Here's how the part is built. I have some questions about the finished solid (model axes, mm). Round coordinates to 2 decimals unless told otherwise and drop trailing zeros. Loops run counter-clockwise (first coordinate to the right, second up) from the corner with the lowest first, then second, coordinate; pieces in that order, holes last. Notation, with made-up numbers: M 36.25,20.25 L 68.25,20.25 A16 ccw 68.25,49.25 Z; hole C 50,74.5 d3. An arc over 180 degrees is marked long. Use a Markdown table: item, result.
from build123d import *

# Parameters (mm, degrees)
SKETCH_1_R             = 5
EXTRUDE_1_DEPTH        = 2.4
SKETCH_2_R             = 4
EXTRUDE_2_DEPTH        = 4.8
EXTRUDE_START          = 0.5
SKETCH_3_R             = 4
EXTRUDE_3_DEPTH        = 0.5
FILLET_1_R             = 0.5
SKETCH_5_R             = 1.5
CUT_EXTRUDE_1_DEPTH    = 0.5
SKETCH_6_W             = 0.3
SKETCH_6_H             = 0.7
SKETCH_8_W             = 0.4
SKETCH_8_H             = 0.2
EXTRUDE_5_DEPTH        = 3.5
FILLET_2_R             = 1
FILLET_3_R             = 0.25
FILLET_2_OF_MIRROR_2_R = 1
FILLET_3_OF_MIRROR_2_R = 0.25


# Read off the part's stored shape, not the designer's step: Зеркальное отражение3
with BuildPart() as part:
    # Эскиз1 → Бобышка-Вытянуть1 (new body)
    with BuildSketch(Plane(origin=(0, 0, 0), x_dir=(1, 0, 0), z_dir=(0, 1, 0))):
        with Locations(Location((0, 0, 0), (0, 0, 270))):
            Circle(SKETCH_1_R)
    extrude(amount=EXTRUDE_1_DEPTH)

    # Эскиз2 → Бобышка-Вытянуть2 (add)
    with BuildSketch(Plane.XZ):
        with Locations(Location((0, 0, 0), (0, 0, 270))):
            Circle(SKETCH_2_R)
    extrude(amount=EXTRUDE_2_DEPTH)

    # Эскиз3 → Бобышка-Вытянуть3 (add)
    with BuildSketch(Plane(origin=(0, 2.4, 0), x_dir=(1, 0, 0), z_dir=(0, 1, 0)).offset(EXTRUDE_START)):
        with Locations(Location((0, 0, 0), (0, 0, 90))):
            Circle(SKETCH_3_R)
    extrude(amount=-EXTRUDE_3_DEPTH)

    # Скругление1
    fillet_1_edges = [part.edges().sort_by_distance(p)[0] for p in [
        (0, 2.9, 4),
    ]]
    fillet(fillet_1_edges, radius=FILLET_1_R - 0.0001)  # a hair under: the kernel refuses the full size

    # Эскиз5 → Вырез-Вытянуть1 (cut)
    with BuildSketch(Plane(origin=(0, 2.9, 0), x_dir=(1, 0, 0), z_dir=(0, 1, 0))):
        with Locations(Location((0, 0, 0), (0, 0, 270))):
            Circle(SKETCH_5_R)
    extrude(amount=-CUT_EXTRUDE_1_DEPTH, mode=Mode.SUBTRACT)

    # По траектории4: sweep along a curve in space
    with BuildLine() as sweep_4_path:
        Line((-3.25, -4.8, 2.25), (-3.25, -5.459878122, 2.25))
        Line((-3.25, -5.459878122, 2.25), (-3.724056905, -7.065490817, 2.25))
        Line((-3.724056905, -7.065490817, 2.25), (-3.4, -7.733693766, 2.25))
        Line((-3.4, -7.733693766, 2.25), (-3.4, -8.3, 2.25))
    # Эскиз6 → По траектории4 (sweep)
    with BuildSketch(Plane(origin=(0, -4.8, -4.8), x_dir=(-1, 0, 0), z_dir=(0, 1, 0))):
        with Locations((3.25, 7.05)):
            Rectangle(SKETCH_6_W, SKETCH_6_H)
    sweep_4 = sweep(path=sweep_4_path.line, transition=Transition.RIGHT)

    # Эскиз8 → Бобышка-Вытянуть5 (add)
    with BuildSketch(Plane(origin=(0, -4.8, 9.6), x_dir=(1, 0, 0), z_dir=(0, 1, 0))):
        with Locations((0, 12.5)):
            Rectangle(SKETCH_8_W, SKETCH_8_H)
        with Locations((0, 6.7)):
            Rectangle(SKETCH_8_W, SKETCH_8_H)
    extrude(amount=-EXTRUDE_5_DEPTH)

    # Скругление2
    fillet_2_edges = [part.edges().sort_by_distance(p)[0] for p in [
        (-3.25, -7.699240124, 2.25),
        (-3.55, -7.768147407, 2.25),
        (-3.884358836, -7.078701954, 2.25),
        (-3.563754975, -7.052279681, 2.25),
        (-3.4, -5.438197011, 2.25),
        (-3.1, -5.481559233, 2.25),
    ]]
    fillet(fillet_2_edges, radius=FILLET_2_R)

    # Скругление3
    fillet_3_edges = [part.edges().sort_by_distance(p)[0] for p in [
        (-3.4, -8.3, 1.9),
        (-3.4, -8.3, 2.6),
    ]]
    fillet(fillet_3_edges, radius=FILLET_3_R)

    # Зеркальное отражение2: По траектории4 across plane
    add(sweep_4.mirror(Plane(origin=(0, 0, 0), x_dir=(0, 0, 1), z_dir=(1, 0, 0))))

    # Скругление2 of Зеркальное отражение2
    fillet_2_of_mirror_2_edges = [part.edges().sort_by_distance(p)[0] for p in [
        (3.25, -7.699240124, 2.25),
        (3.55, -7.768147407, 2.25),
        (3.884358836, -7.078701954, 2.25),
        (3.563754975, -7.052279681, 2.25),
        (3.4, -5.438197011, 2.25),
        (3.1, -5.481559233, 2.25),
    ]]
    fillet(fillet_2_of_mirror_2_edges, radius=FILLET_2_OF_MIRROR_2_R)

    # Скругление3 of Зеркальное отражение2
    fillet_3_of_mirror_2_edges = [part.edges().sort_by_distance(p)[0] for p in [
        (3.4, -8.3, 1.9),
        (3.4, -8.3, 2.6),
    ]]
    fillet(fillet_3_of_mirror_2_edges, radius=FILLET_3_OF_MIRROR_2_R)

    # Зеркальное отражение3: part across plane


with BuildPart() as part_1:
    add(part.part)
    add(part.part.mirror(Plane.XY))


solid = part_1.part
1. Imagine slicing it at D-D, the plane y = 0.5. Write out the boundary of the cut face in (x, z), then the cut area to 3 significant figures.
Answer sheet:
| item | result |
|---|---|
| outline | C 0,0 d10 |
| area | 78.5 mm2 |
2. I need wall thicknesses on probe 1 along Y at (x, z) = (1.75, 2); probe 2 along Y at (x, z) = (0, 0.75); probe 3 along X at (y, z) = (2.75, 0). Which ranges of each line are inside material? Lowest first, please. Write a range as from..to.
Answer sheet:
| item | result |
|---|---|
| probe 1 | -4.8..2.9 |
| probe 2 | -4.8..2.4 |
| probe 3 | -3.86..-1.5, 1.5..3.86 |
3. For pin 1 Ø1.5 at (x, y) = (3, -3.5) entering from -Z; pin 2 Ø0.9 at (x, z) = (0, 0.5) entering from +Y; pin 3 Ø1 at (y, z) = (1, 1.5) entering from -X, each with a flat end and sliding along its axis, tell me the tip position at first contact or that it passes through.
Answer sheet:
| item | result |
|---|---|
| pin 1 | z = -3.31 |
| pin 2 | y = 2.4 |
| pin 3 | x = -4.9 |
4. Imagine slicing it at C-C, the plane y = -2.5. Write out the boundary of the cut face in (x, z), then the cut area to 3 significant figures.
Answer sheet:
| item | result |
|---|---|
| outline | C 0,0 d8 |
| area | 50.3 mm2 |
5. We'd pull the mould along Z, two halves only. Please class faces 1 (the face through (-4.88, 1.18, -1.08)), 2 (the face through (2, 2.9, 0)), 3 (the face through (0.45, 2.65, 1.43)): +Z half, -Z half, draft (parallel to the pull), parting line (faces both ways), or undercut.
Answer sheet:
| item | result |
|---|---|
| face 1 | parting line |
| face 2 | draft |
| face 3 | undercut |
